Autodesk Fusion 360 part; units mm, degrees
sketch "Sketch1" plane through (0, 0, 0) normal (0, 0, 1) x (1, 0, 0)
  line L0 (-5, 5) -> (35, 5)
  line L1 (35, 5) -> (35, -5)
  line L2 (35, -5) -> (-5, -5)
  line L3 (-5, -5) -> (-5, 5)
  arc A0 (-3, 0) -> (3, 0) centre (0, 0) ccw
  arc A1 (-3, 3.7) -> (-3, 4.3) centre (-3, 4) ccw
  arc A2 (3, 4.3) -> (3, 3.7) centre (3, 4) ccw
  line L4 (-3, 0) -> (-3, 3.7)
  line L5 (-3, 4.3) -> (-3, 5)
  line L6 (3, 0) -> (3, 3.7)
  line L7 (3, 4.3) -> (3, 5)
  line L8 (4.5, 4.3) -> (4.5, 5)
  arc A3 (4.5, 3.7) -> (4.5, 4.3) centre (4.5, 4) ccw
  line L9 (4.5, 0) -> (4.5, 3.7)
  arc A4 (4.5, 0) -> (10.5, 0) centre (7.5, 0) ccw
  line L10 (10.5, 0) -> (10.5, 3.7)
  arc A5 (10.5, 4.3) -> (10.5, 3.7) centre (10.5, 4) ccw
  line L11 (10.5, 4.3) -> (10.5, 5)
  line L12 (12, 4.3) -> (12, 5)
  arc A6 (12, 3.7) -> (12, 4.3) centre (12, 4) ccw
  line L13 (12, 0) -> (12, 3.7)
  arc A7 (12, 0) -> (18, 0) centre (15, 0) ccw
  line L14 (18, 0) -> (18, 3.7)
  arc A8 (18, 4.3) -> (18, 3.7) centre (18, 4) ccw
  line L15 (18, 4.3) -> (18, 5)
  line L16 (19.5, 4.3) -> (19.5, 5)
  arc A9 (19.5, 3.7) -> (19.5, 4.3) centre (19.5, 4) ccw
  line L17 (19.5, 0) -> (19.5, 3.7)
  arc A10 (19.5, 0) -> (25.5, 0) centre (22.5, 0) ccw
  line L18 (25.5, 0) -> (25.5, 3.7)
  arc A11 (25.5, 4.3) -> (25.5, 3.7) centre (25.5, 4) ccw
  line L19 (25.5, 4.3) -> (25.5, 5)
  line L20 (27, 4.3) -> (27, 5)
  arc A12 (27, 3.7) -> (27, 4.3) centre (27, 4) ccw
  line L21 (27, 0) -> (27, 3.7)
  arc A13 (27, 0) -> (33, 0) centre (30, 0) ccw
  line L22 (33, 0) -> (33, 3.7)
  arc A14 (33, 4.3) -> (33, 3.7) centre (33, 4) ccw
  line L23 (33, 4.3) -> (33, 5)
  line L24 (39, 5.5) -> (-5, 5.5)
  line L25 (-5, 5.5) -> (-5, 7.5) construction
  line L26 (-5, 7.5) -> (39, 7.5)
  line L27 (39, 7.5) -> (39, 5.5) construction
  line L28 (-13.1667, -0.8333) -> (-8.1667, -0.8333)
  line L29 (-13.1667, 0.1667) -> (-8.1667, 0.1667)
  line L30 (-13.1667, 2.3333) -> (-8.1667, 2.3333)
  line L31 (-13.1667, 3.3333) -> (-8.1667, 3.3333)
  line L32 (-13.4161, -3.985) -> (-5, -5)
  line L33 (-13.1667, 5.5) -> (-5, 5.5)
  line L34 (-13.1667, -3) -> (-5, -3)
  line L35 (-13.4161, 6.485) -> (-5, 7.5)
  arc A15 (-13.1667, 5.5) -> (-13.1667, 3.3333) centre (-13.1667, 4.4167) ccw
  arc A16 (-8.1667, 0.1667) -> (-8.1667, 2.3333) centre (-8.1667, 1.25) ccw
  arc A17 (-13.1667, -0.8333) -> (-13.1667, -3) centre (-13.1667, -1.9167) ccw
  arc A18 (-13.1667, 0.1667) -> (-13.4161, -3.985) centre (-13.1667, -1.9167) ccw
  arc A19 (-8.1667, -0.8333) -> (-8.1667, 3.3333) centre (-8.1667, 1.25) ccw
  arc A20 (-13.4161, 6.485) -> (-13.1667, 2.3333) centre (-13.1667, 4.4167) ccw
  line L36 (39, 7.5) -> (46.5175, 10.2362)
  line L37 (46.5175, 10.2362) -> (47.2016, 8.3568) construction
  arc A21 (47.2016, 8.3568) -> (46.5175, 10.2362) centre (46.8596, 9.2965) ccw
  line L38 (39, 5.5) -> (47.2016, 8.3568)
  line L39 (39, 5.5) -> (37, 5.5) construction
  line L40 (37, 5.5) -> (37, -1)
  line L41 (37, -1) -> (39, -1)
  line L42 (39, -1) -> (39, 5.5)
  line L43 (35, 2) -> (36.0955, 2)
  line L44 (37, 1.75) -> (35.9211, 1.75)
  line L45 (35.7017, 1.3803) -> (37, -1)
  line L46 (36.3191, 2.3618) -> (35, 5)
  arc A22 (35.9211, 1.75) -> (35.7017, 1.3803) centre (35.9211, 1.5) ccw
  arc A23 (36.0955, 2) -> (36.3191, 2.3618) centre (36.0955, 2.25) ccw
  point P0 (36.5, 2)
  point P1 (35.5, 1.75)
  dimension "d5" = 6
  dimension "d11" = 5
  dimension "d12" = 5
  dimension "d13" = 5
  dimension "d14" = 35
  dimension "d15" = 0.6
  dimension "d16" = 1
  dimension "d17" = 0.6
  dimension "d18" = 1
  dimension "d21" = 7.5
  dimension "d22" = 0
  dimension "d23" = 2
  dimension "d24" = 0.5
  dimension "d25" = 40
  dimension "d26" = 44
  dimension "d28" = 2.1667
  dimension "d29" = 2.1667
  dimension "d30" = 2.1667
  dimension "d31" = 3.0833
  dimension "d33" = 3.1667
  dimension "d34" = 3.1667
  dimension "d35" = 8.1667
  dimension "d36" = 8.1667
  dimension "d37" = 3.1667
  dimension "d38" = 4.1667
  dimension "d39" = 4.1667
  dimension "d40" = 4.1667
  dimension "d41" = 8
  dimension "d43" = 160
  dimension "d45" = 2
  dimension "d46" = 90
  dimension "d48" = 2
  dimension "d49" = 6.5
  dimension "d50" = 1.5
  dimension "d51" = 3
  dimension "d52" = 1.5
  dimension "d53" = 2.75
  dimension "d55" = 0.25
  dimension "d56" = 0.25
extrude "Extrude1" add sketch "Sketch1" along normal blind 15 contours L0 L1 L2 L3 A0 A1 A2 L4 L5 L6 L7 L8 A3 L9 A4 L10 A5 L11 L12 A6 L13 A7 L14 A8 L15 L16 A9 L17 A10 L18 A11 L19 L20 A12 L21 A13 L22 A14 L23 | L3 L24 L26 L28 L29 L30 L31 L32 L33 L34 L35 A15 A16 A17 A18 A19 A20 L36 A21 L38 | L1 L43 L46 A23 | L24 L40 L41 L42 | L40 L44 L45 A22
sketch "Sketch2" plane through (0, -5, 0) normal (0, -1, 0) x (1, 0, 0)
  line L0 (-5, 0) -> (35, 0)
  line L1 (35, 0) -> (35, 15)
  line L2 (35, 15) -> (-5, 15)
  line L3 (-5, 15) -> (-5, 0)
  circle A0 centre (15, 7.5) radius 1.75
  line L4 (-5, 15) -> (35, 0) construction
  line L5 (-5, 0) -> (35, 15) construction
  circle A1 centre (15, 7.5) radius 3.5
  dimension "d60" = 3.5
  dimension "d63" = 7
extrude "Extrude2" cut sketch "Sketch2" against normal blind 5 contours A0
extrude "Extrude3" cut sketch "Sketch2" along normal blind -2 and the other way blind 10 contours A1
chamfer "Chamfer1" distance 1.75 angle 45 1 edges at (13.3684, -3, 8.1328)
equation "Diameter = 6 mm"
equation "HolesSpacing = 1.5 mm"
equation "NotchSize = 0.3 mm"
equation "d5 = Diameter"
equation "Thickness = 2 mm"
equation "d11 = Diameter / 2 + Thickness"
equation "d12 = Diameter / 2 + Thickness"
equation "d13 = Diameter / 2 + Thickness"
equation "d14 = Linear Dimension-5"
equation "d15 = NotchSize * 2"
equation "d16 = Thickness / 2"
equation "d17 = NotchSize * 2"
equation "d18 = Thickness / 2"
equation "d21 = Diameter + HolesSpacing"
equation "d23 = Thickness"
equation "d24 = Spacing"
equation "d26 = d25 + Thickness * 2"
equation "d28 = d30"
equation "d29 = d30"
equation "d30 = ( Thickness + Diameter + Spacing - Thickness ) / 3"
equation "d31 = d30 / 2 + Thickness"
equation "d33 = d30 + Thickness / 2"
equation "d34 = d30 + Thickness / 2"
equation "d35 = d30 + Diameter"
equation "d36 = d30 + Diameter"
equation "d37 = d30 + Thickness / 2"
equation "d38 = d30 + Thickness"
equation "d39 = d30 + Thickness"
equation "d40 = d30 + Thickness"
equation "d41 = Diameter + Thickness"
equation "d45 = Thickness"
equation "Spacing = 0.5 mm"
equation "d48 = Thickness"
equation "d49 = Diameter + Spacing"
equation "d50 = Thickness * 3 / 4"
equation "d51 = Diameter / 2"
equation "d52 = Thickness * 3 / 4"
equation "d53 = Diameter / 2 - Spacing / 2"
equation "Fillet = 0.25 mm"
equation "d55 = Fillet"
equation "d56 = Fillet"
equation "d57 = Width"
equation "Width = 15 mm"
equation "d60 = ScrewThread"
equation "ScrewThread = 3.5 mm"
equation "ScrewHead = 7 mm"
equation "d63 = ScrewHead"
equation "d64 = -Thickness - Diameter / 2"
equation "d68 = 2 * Thickness + Diameter"
equation "d70 = Thickness * 3.5 / 4"
The model under review builds one solid part; all positions refer to its coordinate system, in mm. A direction names the side the tool comes from. Give positions to 0.01 mm unless a question says otherwise; leave off trailing zeros. Loops run counter-clockwise (first coordinate to the right, second up) from the corner with the lowest first, then second, coordinate; pieces in that order, holes last. Notation, with made-up numbers: (-34.5, -29.75) - (22.5, -29.75) arc R24 ccw to (22.5, 8.25) - close; hole circle Ø11 at (89.25, 2). An arc over 180 degrees is marked (long way). Answer as a JSON object with one key per item and string values.
Q1. To check wall thickness, follow line 1 along Z through (x, y) = (15, -4.9); line 2 along Y through (x, z) = (-4, 10); line 3 along Y through (x, z) = (-9.5, 5.25). State the ranges of each line that lie inside material, in increasing order.
Worked out:
{"line 1": "z = 0 to 5.75, 9.25 to 15", "line 2": "y = -5 to 5, 5.5 to 7.5", "line 3": "y = -4.46 to -3, -0.83 to 0.17, 2.33 to 3.33, 5.5 to 6.96"}
Q2. Mouldability with a two-part tool opening along X and no side actions: class faces 1 (the flat face through (-4, 5, 7)), 2 (the flat face through (-11, 3.333, 7)), 3 (the cylindrical face through (-15.243, 4.248, 7.395)), 4 (the flat face through (11, 2, 15)) as +X half, -X half, draft (parallel to the pull), parting line (faces both ways), or undercut.
Worked out:
{"face 1": "undercut", "face 2": "undercut", "face 3": "-X half", "face 4": "draft"}
Q3. Add section A-A on x = 7.5. State the section outline as (y, z) points.
Worked out:
{"outline": "(-5, 0) - (-3, 0) - (-3, 15) - (-5, 15) - close; (5.5, 0) - (7.5, 0) - (7.5, 15) - (5.5, 15) - close"}
Q4. For faces 5 (the flat face through (36.34, 0.21, 7.4)), 6 (the flat face through (38, -1, 7)), 7 (the cylindrical face through (-7.084, 1.274, 7.395)), 8 (the cylindrical face through (15, -3, 2)), 9 (the conical face through (16.72, -4.64, 8.21)), list the 3-axis set-ups (+Z, -Z, +X, -X, +Y, -Y) from which the entire face can be reached by the end or side of a thin tool; tool diameter is ignored.
Worked out:
{"face 5": "+Z, -Z, -Y", "face 6": "+Z, -Z, +X, -Y", "face 7": "+Z, -Z, -X", "face 8": "+Z, -Z", "face 9": "none"}
Q5. Insertion check: pin 1 (3 mm diameter, centred on y = 2.5, z = 9.5, fed in from -X); pin 2 (2 mm diameter, centred on x = 19.5, z = 8.5, fed in from +Y); pin 3 (2.5 mm diameter, centred on x = -9, z = 6, fed in from +Y); pin 4 (4 mm diameter, centred on x = 30.5, y = 2.5, fed in from -Z). Each pin has a flat end and moves straight along its axis. Give the tip position at first contact, or say it passes through.
Worked out:
{"pin 1": "stops at x = -15.21", "pin 2": "stops at y = 7.5", "pin 3": "stops at y = 7.17", "pin 4": "passes through"}
